Geometry check sheet. Reference: the model listing, model coordinates, mm. A direction names the side the tool comes from. Give positions to 0.01 mm unless a question says otherwise; leave off trailing zeros. Write each loop counter-clockwise with the first axis right and the second up, starting at its lowest first coordinate (ties: lowest second). Pieces come first, ordered by that corner, then holes. Notation, with made-up numbers: (82, 8) -> (87, 8) arc R20 ccw to (87, 13) -> close; hole circle Ø1 at (15.5, 39.5). An arc over 180 degrees is marked (long way). Write item = value, one per line. Start each with the question number.
1. Mould release check, pull along X, two halves, no side actions. Record for faces 1 (the flat face through (87, 53, -450)), 2 (the flat face through (74.235, 53, -460)), 3 (the flat face through (-100, 11, -443)): pulls with the +X half, pulls with the -X half, needs draft (parallel to the pull), parting line crosses it, or undercut.
2. Cross-section at B-B, the plane x = -26. Record the cut outline in (y, z).
3. Thickness scan on line 1 along Y through (x, z) = (68, -6); line 2 along Z through (x, y) = (16.5, 64); line 3 along Z through (x, y) = (80.5, 53.5). Record the ranges inside material, lowest first.
4. Cross-section at C-C, the plane z = -719. Record the cut outline in (x, y).
5. Cross-section at A-A, the plane y = 50. Record the cut outline in (x, z).
6. Depth check by flat-ended pin: P1, Ø8.5, axis at x = -81, y = 48.5, coming from the +Z side; P2, Ø20.5, axis at x = 88.5, y = 59, coming from the -Z side. Enter the tip coordinate at first touch or a pass-through.
7. Set-up check for faces 4 (the flat face through (100, 11, -443)), 5 (the flat face through (87, 53, -470)), 6 (the flat face through (-86, 53, -450)): record each of +Z, -Z, +X, -X, +Y, -Y from which the full face is reachable in a straight line by a thin tool's end or side.
```python
from build123d import *

# Parameters (mm, degrees)
ESQUISSE3_W             = 1000
ESQUISSE3_H             = 50
BOSS_EXTRU_2_DEPTH      = 100
BOSS_EXTRU_2_DEPTH_BACK = 100
ESQUISSE4_W             = 27.549124878
ESQUISSE4_H             = 20
ESQUISSE4_W_2           = 25.7645404
BOSS_EXTRU_4_DEPTH      = 30
ESQUISSE7_R             = 3.448131388
BOSS_EXTRU_5_DEPTH      = 157
BOSS_EXTRU_5_DEPTH_BACK = 15


with BuildPart() as part:
    # Esquisse3 → Boss.-Extru.2 (new body, two sides)
    with BuildSketch(Plane(origin=(0, 0, 0), x_dir=(0, 0, -1), z_dir=(1, 0, 0))) as boss_extru_2_sk:
        with Locations((450, 13.600000315)):
            Rectangle(ESQUISSE3_W, ESQUISSE3_H)
    extrude(amount=BOSS_EXTRU_2_DEPTH)
    extrude(boss_extru_2_sk.sketch, amount=-BOSS_EXTRU_2_DEPTH_BACK)

    # Esquisse4 → Boss.-Extru.4 (add)
    with BuildSketch(Plane(origin=(0, 38.600000315, 0), x_dir=(1, 0, 0), z_dir=(0, 1, 0))):
        with Locations((-86.225437561, 460)):
            Rectangle(ESQUISSE4_W, ESQUISSE4_H)
        with Locations((87.1177298, 460)):
            Rectangle(ESQUISSE4_W_2, ESQUISSE4_H)
    extrude(amount=BOSS_EXTRU_4_DEPTH)

    # Esquisse7 → Boss.-Extru.5 (add, two sides)
    with BuildSketch(Plane(origin=(-72.450875122, 0, 0), x_dir=(0, 0, -1), z_dir=(1, 0, 0))) as boss_extru_5_sk:
        with Locations((458.615528394, 65.151868928)):
            Circle(ESQUISSE7_R)
    extrude(amount=BOSS_EXTRU_5_DEPTH)
    extrude(boss_extru_5_sk.sketch, amount=-BOSS_EXTRU_5_DEPTH_BACK)


solid = part.part
```
Answers:
q1.face_1 = needs draft
q1.face_2 = undercut
q1.face_3 = pulls with the -X half
q2.outline = (-11.4, -950) -> (38.6, -950) -> (38.6, 50) -> (-11.4, 50) -> close; circle Ø6.9 at (65.15, -458.62)
q3.line_1 = -11.4 to 38.6
q3.line_2 = -461.87 to -455.37
q3.line_3 = -470 to -450
q4.outline = (-100, -11.4) -> (100, -11.4) -> (100, 38.6) -> (-100, 38.6) -> close
q5.outline = (-100, -470) -> (-72.45, -470) -> (-72.45, -450) -> (-100, -450) -> close; (74.24, -470) -> (100, -470) -> (100, -450) -> (74.24, -450) -> close
q6.P1 = -450
q6.P2 = -470
q7.face_4 = +Z, -Z, +X, +Y, -Y
q7.face_5 = -Z, +X, -X, +Y
q7.face_6 = +Z, +X, -X, +Y
